Source: CAD feature listing. Evaluate the final solid. Frame: model axes, mm. A direction names the side the tool comes from. Give positions to 0.01 mm unless a question says otherwise; leave off trailing zeros. Order: outer loops, then holes, each group sorted by start corner. A loop starts at its lowest first (then second) coordinate and runs counter-clockwise, first axis right, second up.
1) Section B-B, the plane z = 15.75. Return loops of the section in (x, y), plus the area to 3 significant figures.
2) Section C-C, the plane x = 66. Return loops of the section in (y, z).
3) Section A-A, the plane y = 10. Return loops of the section in (x, z), plus the area to 3 significant figures.
4) Material intervals for line 1 (Y direction, x = 13, z = 15.75), sorted ascending.
5) Draft query along X for faces 3 (the face through (61.546, 10, 13)), 4 (the face through (44, 0, 13)). Return one class per face: released by +X, released by -X, zero draft, split by the parting line, or undercut.
6) First-contact query: P1, Ø2, axis at x = 50, z = 11, coming from the -Y side. Flat tip, straight axial feed; report the tip coordinate or a pass-through.
7) Access query for faces 1 (the face through (54.708, 10, 14)), 2 (the face through (58, 13.47, 13)). Directions: +Z, -Z, +X, -X, +Y, -Y. A direction counts if a zero-diameter tool reaches every point of the face in a straight line with its end or side. Return the directions, or none.
Autodesk Fusion 360 part; units mm, degrees
sketch "Sketch1" plane through (0, 0, 0) normal (0, 1, 0) x (1, 0, 0)
  line L0 (0, 0) -> (88, 0)
  line L1 (88, 0) -> (88, 8.2)
  line L2 (88, 8.2) -> (0, 8.2)
  line L3 (0, 8.2) -> (0, 0)
  dimension "d1" = 88
  dimension "d2" = 8.2
sketch "Sketch2" plane through (0, 12.75, 0) normal (0, 1, 0) x (-1, 0, 0)
  line L0 (0, -8.2) -> (0, 0)
  line L1 (0, 0) -> (-88, 0)
  line L2 (-88, 0) -> (-88, -8.2)
  line L3 (-88, -8.2) -> (0, -8.2)
  line L4 (0, 0) -> (-6.77, 0)
  line L5 (-6.77, 0) -> (-6.77, -8.2)
  line L6 (-6.77, -8.2) -> (0, -8.2)
  line L7 (0, -8.2) -> (0, 0)
  line L8 (-6.77, -8.2) -> (-13.54, -8.2)
  line L9 (-13.54, -8.2) -> (-13.54, 0)
  line L10 (-13.54, 0) -> (-6.77, 0)
  line L11 (-6.77, 0) -> (-6.77, -8.2)
  dimension "d5" = 6.77
  dimension "d6" = 6.77
sketch "Sketch3" plane through (0, 12.75, 0) normal (0, 1, 0) x (-1, 0, 0)
  line L0 (-13.54, -8.2) -> (-13.54, 0)
  line L1 (-13.54, 0) -> (-88, 0)
  line L2 (-88, 0) -> (-88, -8.2)
  line L3 (-88, -8.2) -> (-13.54, -8.2)
  line L4 (-13.54, 0) -> (-20.31, 0)
  line L5 (-20.31, 0) -> (-20.31, -8.2)
  line L6 (-20.31, -8.2) -> (-13.54, -8.2)
  line L7 (-13.54, -8.2) -> (-13.54, 0)
  line L8 (-20.31, -8.2) -> (-27.08, -8.2)
  line L9 (-27.08, -8.2) -> (-27.08, 0)
  line L10 (-27.08, 0) -> (-20.31, 0)
  line L11 (-20.31, 0) -> (-20.31, -8.2)
  dimension "d9" = 6.77
  dimension "d10" = 6.77
sketch "Sketch4" plane through (0, 12.75, 0) normal (0, 1, 0) x (-1, 0, 0)
  line L0 (-27.08, -8.2) -> (-27.08, 0)
  line L1 (-27.08, 0) -> (-88, 0)
  line L2 (-88, 0) -> (-88, -8.2)
  line L3 (-88, -8.2) -> (-27.08, -8.2)
  line L4 (-27.08, 0) -> (-33.85, 0)
  line L5 (-33.85, 0) -> (-33.85, -8.2)
  line L6 (-33.85, -8.2) -> (-27.08, -8.2)
  line L7 (-27.08, -8.2) -> (-27.08, 0)
  line L8 (-33.85, -8.2) -> (-40.62, -8.2)
  line L9 (-40.62, -8.2) -> (-40.62, 0)
  line L10 (-40.62, 0) -> (-33.85, 0)
  line L11 (-33.85, 0) -> (-33.85, -8.2)
  dimension "d13" = 6.77
  dimension "d14" = 6.77
sketch "Sketch5" plane through (0, 12.75, 0) normal (0, 1, 0) x (-1, 0, 0)
  line L0 (-40.62, -8.2) -> (-40.62, 0)
  line L1 (-40.62, 0) -> (-88, 0)
  line L2 (-88, 0) -> (-88, -8.2)
  line L3 (-88, -8.2) -> (-40.62, -8.2)
  line L4 (-40.62, 0) -> (-47.39, 0)
  line L5 (-47.39, 0) -> (-47.39, -8.2)
  line L6 (-47.39, -8.2) -> (-40.62, -8.2)
  line L7 (-40.62, -8.2) -> (-40.62, 0)
  line L8 (-47.39, -8.2) -> (-54.16, -8.2)
  line L9 (-54.16, -8.2) -> (-54.16, 0)
  line L10 (-54.16, 0) -> (-47.39, 0)
  line L11 (-47.39, 0) -> (-47.39, -8.2)
  dimension "d17" = 6.77
  dimension "d18" = 6.77
sketch "Sketch6" plane through (0, 12.75, 0) normal (0, 1, 0) x (-1, 0, 0)
  line L0 (-54.16, -8.2) -> (-54.16, 0)
  line L1 (-54.16, 0) -> (-88, 0)
  line L2 (-88, 0) -> (-88, -8.2)
  line L3 (-88, -8.2) -> (-54.16, -8.2)
  line L4 (-54.16, 0) -> (-60.93, 0)
  line L5 (-60.93, 0) -> (-60.93, -8.2)
  line L6 (-60.93, -8.2) -> (-54.16, -8.2)
  line L7 (-54.16, -8.2) -> (-54.16, 0)
  line L8 (-60.93, 0) -> (-67.7, 0)
  line L9 (-67.7, 0) -> (-67.7, -8.2)
  line L10 (-67.7, -8.2) -> (-60.93, -8.2)
  line L11 (-60.93, -8.2) -> (-60.93, 0)
  dimension "d21" = 6.77
  dimension "d22" = 6.77
sketch "Sketch7" plane through (0, 12.75, 0) normal (0, 1, 0) x (-1, 0, 0)
  line L0 (-67.7, -8.2) -> (-67.7, 0)
  line L1 (-67.7, 0) -> (-88, 0)
  line L2 (-88, 0) -> (-88, -8.2)
  line L3 (-88, -8.2) -> (-67.7, -8.2)
  line L4 (-67.7, 0) -> (-74.47, 0)
  line L5 (-74.47, 0) -> (-74.47, -8.2)
  line L6 (-74.47, -8.2) -> (-67.7, -8.2)
  line L7 (-67.7, -8.2) -> (-67.7, 0)
  line L8 (-74.47, -8.2) -> (-81.24, -8.2)
  line L9 (-81.24, -8.2) -> (-81.24, 0)
  line L10 (-81.24, 0) -> (-74.47, 0)
  line L11 (-74.47, 0) -> (-74.47, -8.2)
  dimension "d25" = 6.77
  dimension "d26" = 6.77
sketch "Sketch8" plane through (0, 0, 0) normal (0, 1, 0) x (1, 0, 0)
sketch "Sketch9" plane through (0, 0, 0) normal (0, 1, 0) x (1, 0, 0)
  line L0 (0, -10) -> (88.9, -10)
  line L1 (88.9, -10) -> (88.9, -17.02)
  line L2 (88.9, -17.02) -> (0, -17.02)
  line L3 (0, -17.02) -> (0, -10)
  dimension "d32" = 88.9
  dimension "d33" = 7.02
extrude "Extrude9" add sketch "Sketch9" along normal blind 13.47
sketch "Sketch10" plane through (0, 13.47, 0) normal (0, 1, 0) x (-1, 0, 0)
  line L0 (0, 17.02) -> (-88.9, 17.02)
  line L1 (-88.9, 17.02) -> (-88.9, 10)
  line L2 (-88.9, 10) -> (0, 10)
  line L3 (0, 10) -> (0, 17.02)
  line L4 (-6.8385, 17.02) -> (-13.6769, 17.02)
  line L5 (-13.6769, 17.02) -> (-13.6769, 10)
  line L6 (-13.6769, 10) -> (-6.8385, 10)
  line L7 (-6.8385, 10) -> (-6.8385, 17.02)
  line L8 (-20.5154, 17.02) -> (-27.3538, 17.02)
  line L9 (-27.3538, 17.02) -> (-27.3538, 10)
  line L10 (-27.3538, 10) -> (-20.5154, 10)
  line L11 (-20.5154, 10) -> (-20.5154, 17.02)
  line L12 (-34.1923, 17.02) -> (-41.0308, 17.02)
  line L13 (-41.0308, 17.02) -> (-41.0308, 10)
  line L14 (-41.0308, 10) -> (-34.1923, 10)
  line L15 (-34.1923, 10) -> (-34.1923, 17.02)
  line L16 (-47.8692, 17.02) -> (-54.7077, 17.02)
  line L17 (-54.7077, 17.02) -> (-54.7077, 10)
  line L18 (-54.7077, 10) -> (-47.8692, 10)
  line L19 (-47.8692, 10) -> (-47.8692, 17.02)
  line L20 (-61.5462, 17.02) -> (-68.3846, 17.02)
  line L21 (-68.3846, 17.02) -> (-68.3846, 10)
  line L22 (-68.3846, 10) -> (-61.5462, 10)
  line L23 (-61.5462, 10) -> (-61.5462, 17.02)
  line L24 (-75.2231, 17.02) -> (-82.0615, 17.02)
  line L25 (-82.0615, 17.02) -> (-82.0615, 10)
  line L26 (-82.0615, 10) -> (-75.2231, 10)
  line L27 (-75.2231, 10) -> (-75.2231, 17.02)
  point P0 (0, 17.02)
  point P1 (-6.8385, 17.02)
  point P2 (-13.6769, 17.02)
  point P3 (-20.5154, 17.02)
  point P4 (-27.3538, 17.02)
  point P5 (-34.1923, 17.02)
  point P6 (-41.0308, 17.02)
  point P7 (-47.8692, 17.02)
  point P8 (-54.7077, 17.02)
  point P9 (-61.5462, 17.02)
  point P10 (-68.3846, 17.02)
  point P11 (-75.2231, 17.02)
  point P12 (-82.0615, 17.02)
  point P13 (-88.9, 17.02)
  dimension "d38" = 88.9
  dimension "d39" = 0
  dimension "d40" = 6.8385
  dimension "d43" = 6.8385
  dimension "d46" = 6.8385
  dimension "d47" = 6.8385
  dimension "d48" = 6.8385
  dimension "d49" = 7.02
  dimension "d50" = 6.8385
extrude "Extrude12" cut sketch "Sketch10" against normal blind 6.5 contours L0 L2 L4 L5 L6 L7
extrude "Extrude11" cut sketch "Sketch10" against normal blind 6.5 contours L0 L2 L4 L5 L6 L7
extrude "Extrude10" cut sketch "Sketch10" against normal blind 6.5 contours L0 L2 L4 L5 L6 L7
extrude "Extrude13" cut sketch "Sketch10" against normal blind 6.5 contours L0 L2 L8 L9 L10 L11
extrude "Extrude14" cut sketch "Sketch10" against normal blind 6.5 contours L0 L2 L12 L13 L14 L15
extrude "Extrude15" cut sketch "Sketch10" against normal blind 6.5 contours L0 L2 L16 L17 L18 L19
extrude "Extrude16" cut sketch "Sketch10" against normal blind 6.5 contours L0 L2 L20 L21 L22 L23
extrude "Extrude17" cut sketch "Sketch10" against normal blind 6.5 contours L0 L2 L24 L25 L26 L27
From the geometry:
1. outline: (0, 0) - (88.9, 0) - (88.9, 13.47) - (82.06, 13.47) - (82.06, 6.97) - (75.22, 6.97) - (75.22, 13.47) - (68.38, 13.47) - (68.38, 6.97) - (61.55, 6.97) - (61.55, 13.47) - (54.71, 13.47) - (54.71, 6.97) - (47.87, 6.97) - (47.87, 13.47) - (41.03, 13.47) - (41.03, 6.97) - (34.19, 6.97) - (34.19, 13.47) - (27.35, 13.47) - (27.35, 6.97) - (20.52, 6.97) - (20.52, 13.47) - (13.68, 13.47) - (13.68, 6.97) - (6.84, 6.97) - (6.84, 13.47) - (0, 13.47) - close
1. area: 931 mm2
2. outline: (0, 10) - (6.97, 10) - (6.97, 17.02) - (0, 17.02) - close
3. outline: (0, 10) - (6.84, 10) - (6.84, 17.02) - (0, 17.02) - close; (13.68, 10) - (20.52, 10) - (20.52, 17.02) - (13.68, 17.02) - close; (27.35, 10) - (34.19, 10) - (34.19, 17.02) - (27.35, 17.02) - close; (41.03, 10) - (47.87, 10) - (47.87, 17.02) - (41.03, 17.02) - close; (54.71, 10) - (61.55, 10) - (61.55, 17.02) - (54.71, 17.02) - close; (68.38, 10) - (75.22, 10) - (75.22, 17.02) - (68.38, 17.02) - close; (82.06, 10) - (88.9, 10) - (88.9, 17.02) - (82.06, 17.02) - close
3. area: 336 mm2
4. line 1: y = 0 to 6.97
5. face 3: undercut
5. face 4: zero draft
6. P1: stops at y = 0
7. face 1: +Z, -Z, +Y
7. face 2: +Z, -Z, +X, -X, +Y
